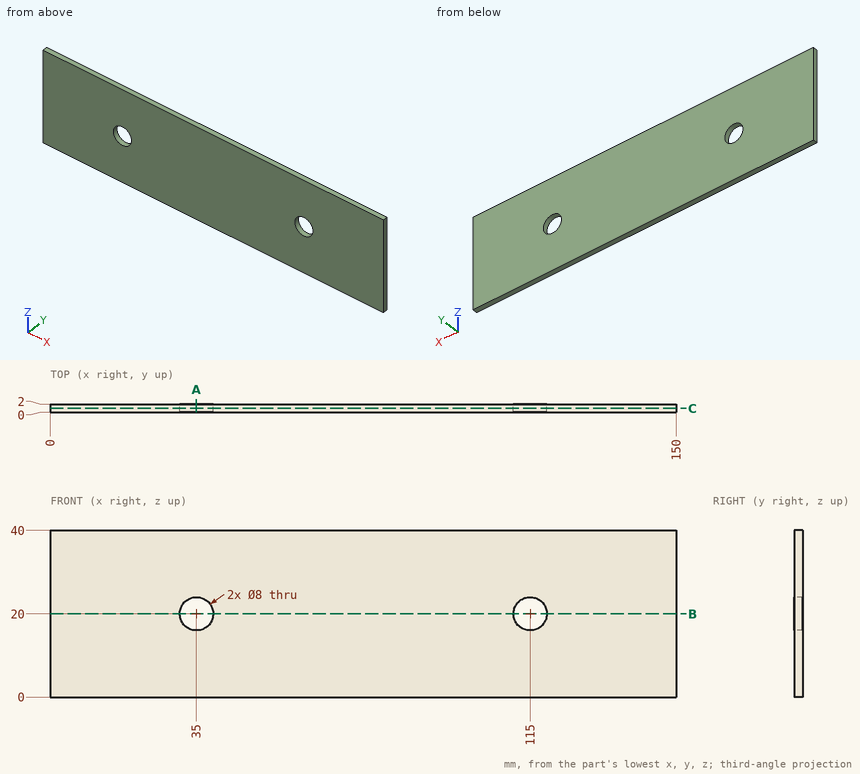
Source: three-view drawing plus pictorial views. Frame: mm from the lowest corner of the part. Coordinates: 2 decimals unless noted, no trailing zeros. Loops run counter-clockwise (first coordinate to the right, second up) from the corner with the lowest first, then second, coordinate; pieces in that order, holes last. Notation, with made-up numbers: (83.5, 31.25) - (91.5, 31.25) arc R10 ccw to (91.5, 41.25) - close; hole circle Ø10 at (-29, 26.5). An arc over 180 degrees is marked (long way). Answer in a Markdown table with one row per item. Add a question column.
Item 1: Contact query for a flat-ended pin moving along its axis: P1, Ø6.5, axis at x = 115, z = 20, coming from the -Y side. Output: stop coordinate, or through.
Item 2: Section query C-C on y = 0.95. Return the cut outline in (x, z), then the cut area to 3 significant figures.
Item 3: Section query B-B on z = 20. Return the cut outline in (x, y), then the cut area to 3 significant figures.
Item 4: Section query A-A on x = 35. Return the cut outline in (y, z).
Item 5: Line query: line 1 along X through (y, z) = (0.55, 20); line 2 along Z through (x, y) = (115, 1.1); line 3 along X through (y, z) = (0.85, 22.5). Output: solid intervals per line, ascending. Write a range as [from, to].
Recorded:
| question | item | result |
|---|---|---|
| 1 | P1 | through |
| 2 | outline | (0, 0) - (150, 0) - (150, 40) - (0, 40) - close; hole circle Ø8 at (35, 20); hole circle Ø8 at (115, 20) |
| 2 | area | 5,900 mm^2 |
| 3 | outline | (0, 0) - (31, 0) - (31, 2) - (0, 2) - close; (39, 0) - (111, 0) - (111, 2) - (39, 2) - close; (119, 0) - (150, 0) - (150, 2) - (119, 2) - close |
| 3 | area | 268 mm^2 |
| 4 | outline | (0, 0) - (2, 0) - (2, 16) - (0, 16) - close; (0, 24) - (2, 24) - (2, 40) - (0, 40) - close |
| 5 | line 1 | [0, 31], [39, 111], [119, 150] |
| 5 | line 2 | [0, 16], [24, 40] |
| 5 | line 3 | [0, 31.88], [38.12, 111.88], [118.12, 150] |
